Source: three-view drawing plus pictorial views. Frame: mm from the lowest corner of the part. A direction names the side the tool comes from. Coordinates: 2 decimals unless noted, no trailing zeros. Order: outer loops, then holes, each group sorted by start corner. A loop starts at its lowest first (then second) coordinate and runs counter-clockwise, first axis right, second up. Notation, with made-up numbers: (49, 77) - (100, 77) arc R22 ccw to (100, 99) - close; hole circle Ø4 at (-17.5, 6.25). An arc over 180 degrees is marked (long way). Use a Markdown table: item, result. Add a question column.
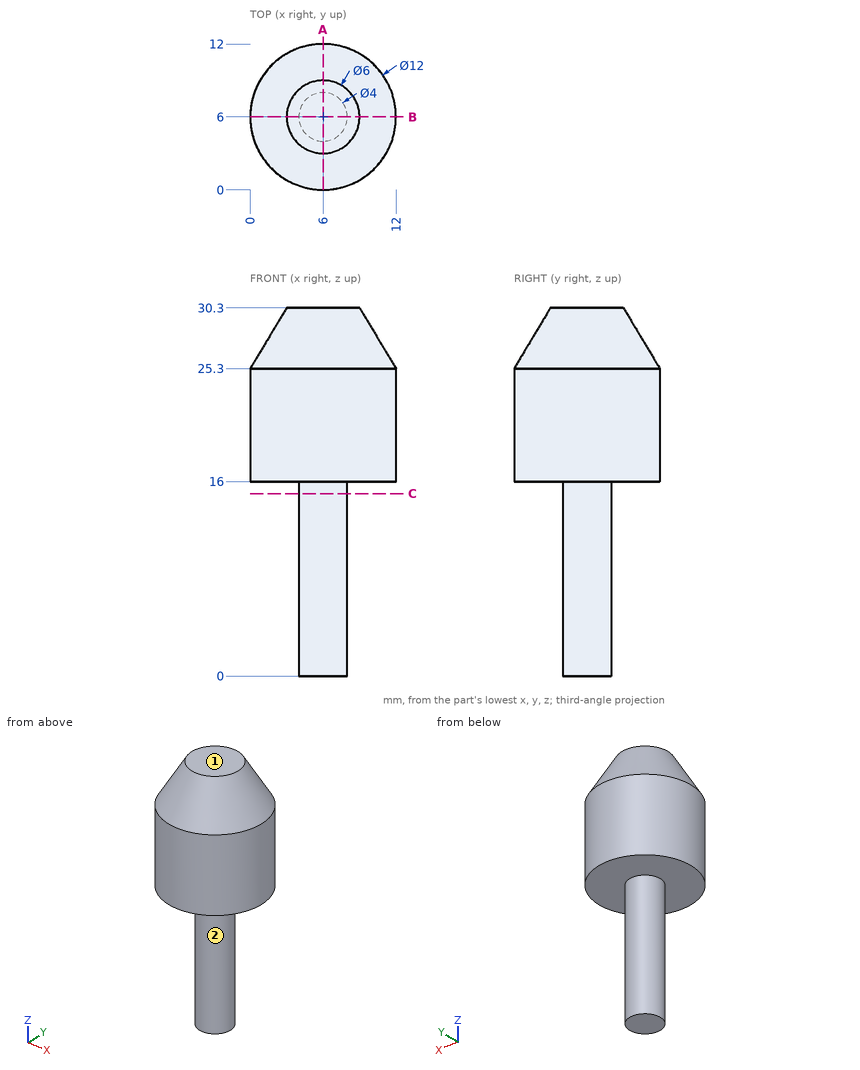
1) Section C-C (z = 15). Return loops of the section in (x, y).
2) Section A-A (x = 6). Return loops of the section in (y, z).
3) Set-up query: the marked faces 1 and 2. Return all of +Z, -Z, +X, -X, +Y, -Y with unobstructed straight access to the full face (end or side cutting, diameter ignored); none if empty.
4) Ray query, line 1 along Z through (x, y) = (3, 2.75); line 2 along Z through (x, y) = (8, 1.75); line 3 along X through (y, z) = (5.5, 19). Return the intervals inside material, ascending.
5) Pin query (flat end, axial travel): pin 1 (4 mm diameter, centred on x = 2.5, z = 17, fed in from -Y); pin 2 (4 mm diameter, centred on x = 6.5, y = 5.5, fed in from -Z); pin 3 (4 mm diameter, centred on y = 2.5, z = 20.5, fed in from -X); pin 4 (1 mm diameter, centred on x = 7.5, y = 9.5, fed in from -Z). Return the tip coordinate at first contact, or that it passes through.
Values follow:
| question | item | result |
|---|---|---|
| 1 | outline | circle Ø4 at (6, 6) |
| 2 | outline | (0, 16) - (4, 16) - (4, 0) - (8, 0) - (8, 16) - (12, 16) - (12, 25.3) - (9, 30.3) - (3, 30.3) - (0, 25.3) - close |
| 3 | face 1 | +Z, +X, -X, +Y, -Y |
| 3 | face 2 | -Z |
| 4 | line 1 | z = 16 to 27.93 |
| 4 | line 2 | z = 16 to 27.47 |
| 4 | line 3 | x = 0.02 to 11.98 |
| 5 | pin 1 | stops at y = 0.19 |
| 5 | pin 2 | stops at z = 0 |
| 5 | pin 3 | stops at x = 0.19 |
| 5 | pin 4 | stops at z = 16 |
